Study the drawing (mm; zero at the part's minimum x, y, z) and answer. A direction names the side the tool comes from. Round coordinates to 2 decimals unless told otherwise and drop trailing zeros. Order: outer loops, then holes, each group sorted by start corner. A loop starts at its lowest first (then second) coordinate and runs counter-clockwise, first axis right, second up. Notation, with made-up numbers: (9, -18.75) -> (31, -18.75) arc R15 ccw to (31, 4.25) -> close; hole circle Ø6 at (82.5, 14). An arc over 180 degrees is marked (long way). Use one line per item in the form item = value.
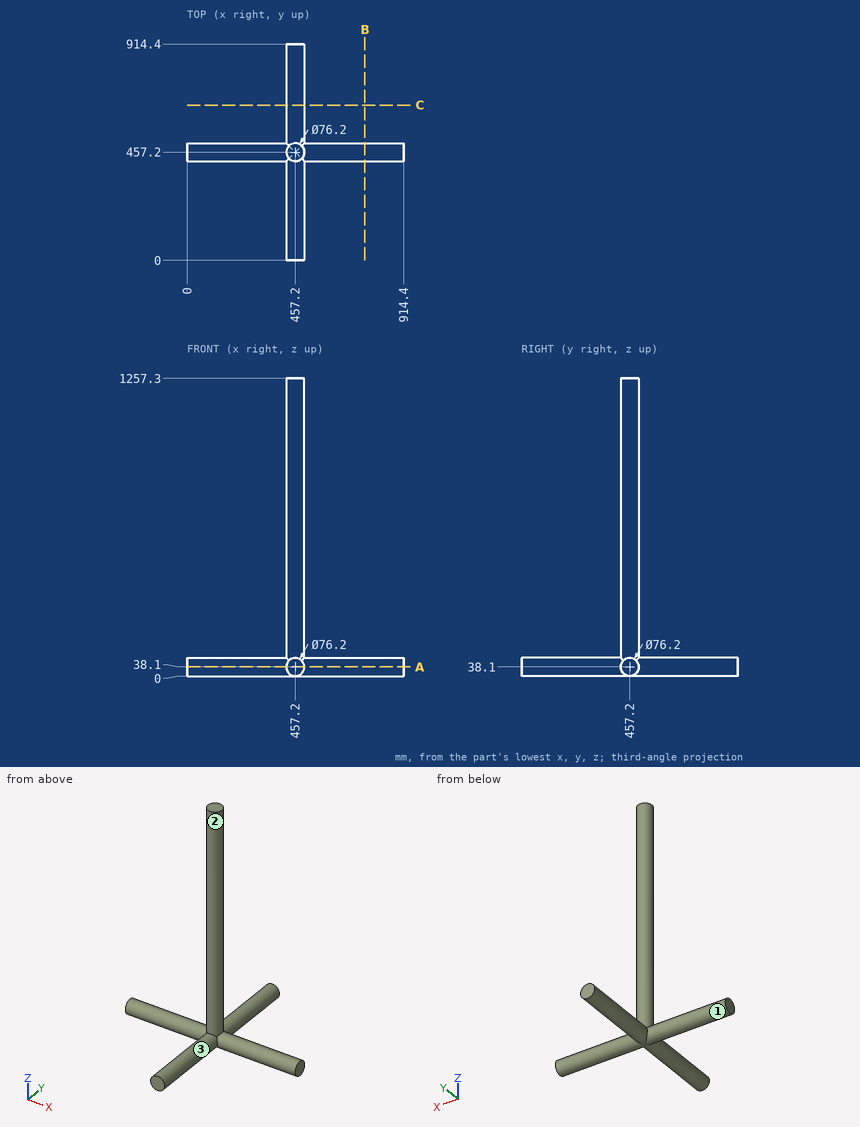
Item 1: The part is cut by section A-A, the plane z = 38.1. Give the vertices of the cut face in (x, y), and give its area (3 significant figures).
Findings:
outline = (0, 419.1) -> (419.1, 419.1) -> (419.1, 0) -> (495.3, 0) -> (495.3, 419.1) -> (914.4, 419.1) -> (914.4, 495.3) -> (495.3, 495.3) -> (495.3, 914.4) -> (419.1, 914.4) -> (419.1, 495.3) -> (0, 495.3) -> close
area = 134,000 mm^2
Item 2: For the marked faces 1, 2 and 3, determine the directions among +Z, -Z, +X, -X, +Y, -Y from which every point of the face is accessible in a straight line to the end or side of a thin tool.
Findings:
face_1 = -X
face_2 = +Z
face_3 = -Y
Item 3: Consider line 1 along Z through (x, y) = (457, 100); line 2 along Z through (x, y) = (463.5, 116); line 3 along X through (y, z) = (434, 919). Determine where each line is inside the solid, lowest interval first.
Findings:
line_1 = 0 to 76.2
line_2 = 0.52 to 75.68
line_3 = 426.98 to 487.42
Item 4: The part is cut by section B-B, the plane x = 751. Give the vertices of the cut face in (y, z), and give its area (3 significant figures).
Findings:
outline = circle Ø76.2 at (457.2, 38.1)
area = 4,560 mm^2
